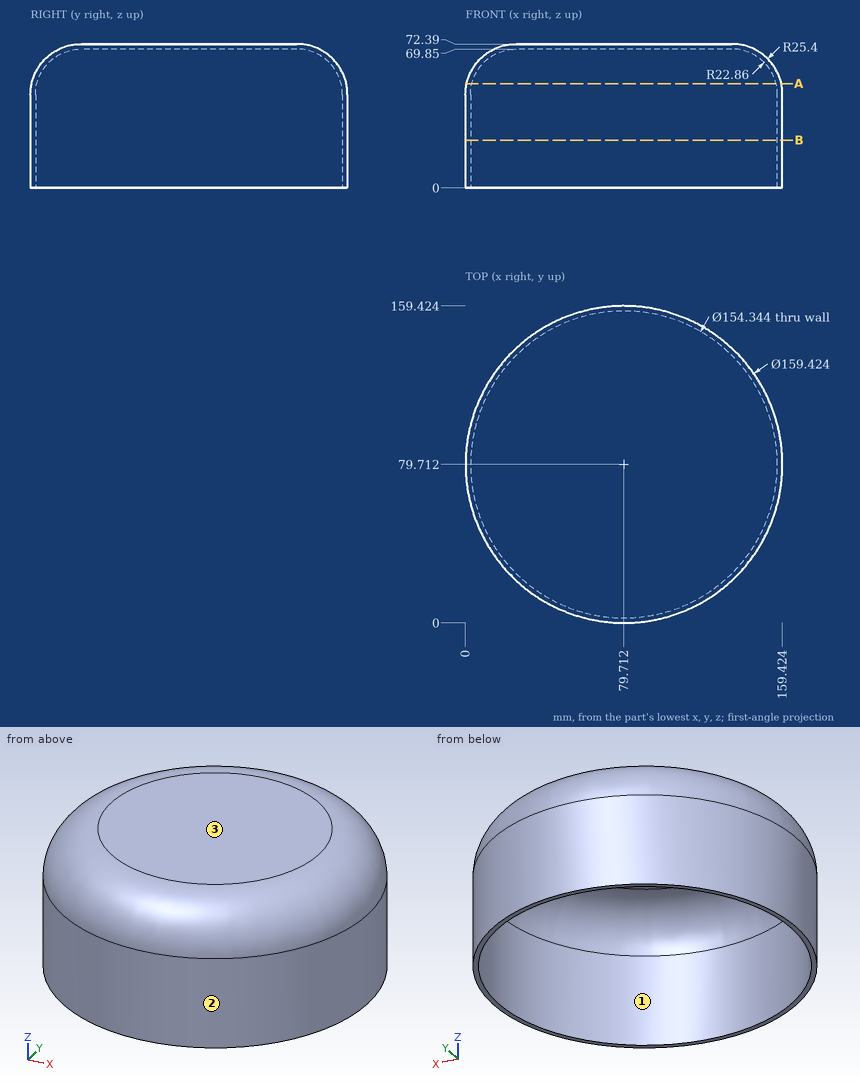
Source: three-view drawing plus pictorial views. Frame: mm from the lowest corner of the part. Round coordinates to 2 decimals unless told otherwise and drop trailing zeros. Order: outer loops, then holes, each group sorted by start corner. A loop starts at its lowest first (then second) coordinate and runs counter-clockwise, first axis right, second up. Notation, with made-up numbers: (-8, 39.25) -> (1, 39.25) arc R28 cw to (1, 64.25) -> close; hole circle Ø2 at (-23.5, 11.25). An arc over 180 degrees is marked (long way). Use CSV: the item, a comma, the result in double quotes. Start each with the question number.
1) Section B-B (z = 24). Return the cut outline in (x, y) (1 decimal).
2) Draft query along X for the marked faces 1, 2 and 3. Return one class per face: +X half, -X half, draft (parallel to the pull), parting line (faces both ways), or undercut.
3) Section A-A (z = 52.5). Return the cut outline in (x, y) (1 decimal).
4) First-contact query: pin 1 Ø12 at (x, y) = (77, 59) entering from -Z; pin 2 Ø8 at (y, z) = (59, 18.5) entering from -X; pin 3 Ø1 at (x, z) = (86, 26.5) entering from +Y. Flat tips, straight axial feed; report the tip coordinate or a pass-through.
5) Material intervals for line 1 along Y through (x, z) = (82, 7); line 2 along X through (y, z) = (128, 16.5) (1 decimal); line 3 along Y through (x, z) = (40.5, 29) (1 decimal), sorted ascending. Write a range as from..to.
Returned:
1,outline,"circle Ø159.4 at (79.7, 79.7); hole circle Ø154.3 at (79.7, 79.7)"
2,face 1,"undercut"
2,face 2,"parting line"
2,face 3,"draft"
3,outline,"circle Ø158.2 at (79.7, 79.7); hole circle Ø153 at (79.7, 79.7)"
4,pin 1,"stops at z = 69.85"
4,pin 2,"stops at x = 1.77"
4,pin 3,"stops at y = 159.21"
5,line 1,"y = 0.03..2.57, 156.85..159.39"
5,line 2,"x = 16.3..19.5, 139.9..143.1"
5,line 3,"y = 10.3..13.2, 146.2..149.1"
